Here's the drawing with two shaded views (mm, measured from the low corner). I have some questions. Give positions to 0.01 mm unless a question says otherwise; leave off trailing zeros. Loops run counter-clockwise (first coordinate to the right, second up) from the corner with the lowest first, then second, coordinate; pieces in that order, holes last. Notation, with made-up numbers: (-35, -34.5) - (6, -34.5) arc R20 cw to (6, -28.5) - close; hole circle Ø9 at (75, 30). An arc over 180 degrees is marked (long way). Use one line per item in the form item = value.
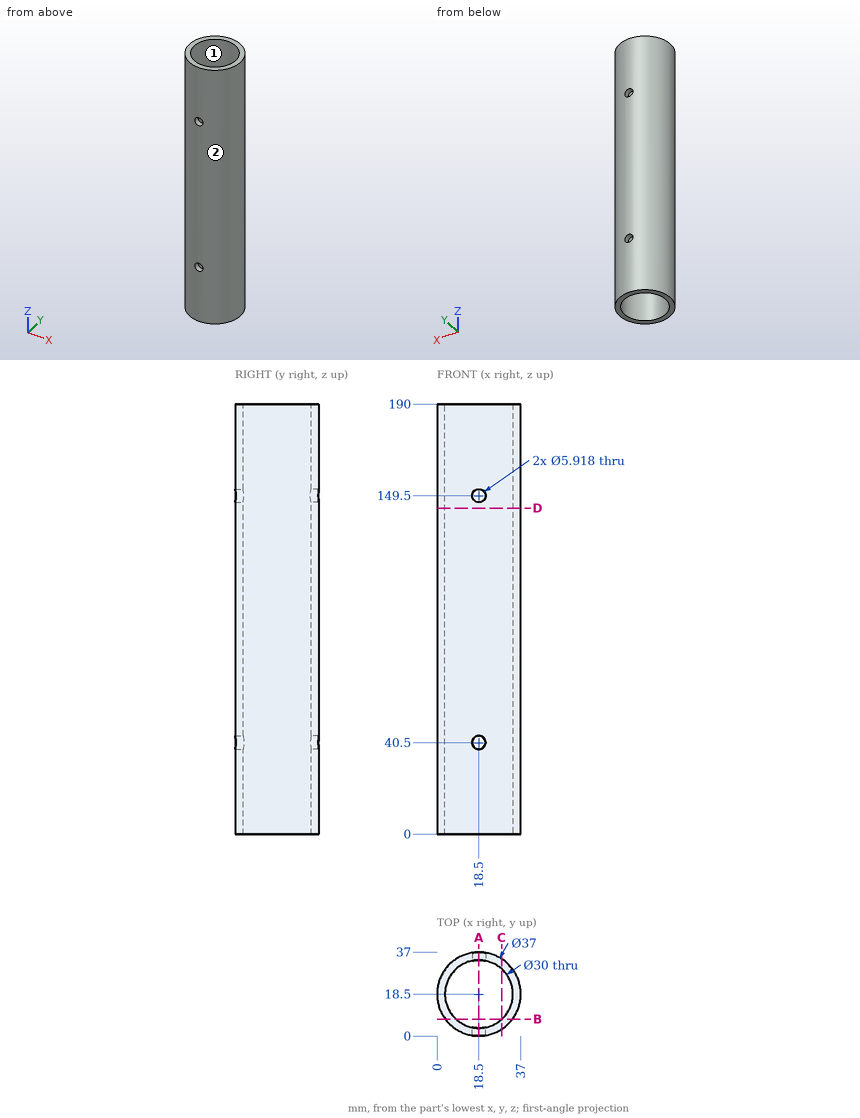
(1) Thinking about a two-plate mould opening in X: for the marked faces 1 and 2, which applies, pulls with the +X half, pulls with the -X half, needs draft (parallel to the pull), parting line crosses it, or undercut?
Geometry says:
face_1 = undercut
face_2 = parting line crosses it
(2) If I drill on probe 1 along Y at (x, z) = (30.5, 142.5); probe 2 along Y at (x, z) = (13, 171) (1 decimal); probe 3 along X at (y, z) = (8.5, 103.5) (1 decimal), over which ranges is the centre line in solid material (lowest first)?
Geometry says:
probe_1 = 4.42 to 9.5, 27.5 to 32.58
probe_2 = 0.8 to 4.5, 32.5 to 36.2
probe_3 = 2.9 to 7.3, 29.7 to 34.1
(3) If we section it at C-C (x = 28.5): List the corners of the cut face in (y, z) for me (1 decimal), plus the area to 3 significant figures.
Geometry says:
outline = (2.9, 0) - (7.3, 0) - (7.3, 190) - (2.9, 190) - close; (29.7, 0) - (34.1, 0) - (34.1, 190) - (29.7, 190) - close
area = 1,670 mm²
(4) If we section it at B-B (y = 7.5): List the corners of the cut face in (x, z) for me (1 decimal), plus the area to 3 significant figures.
Geometry says:
outline = (3.6, 0) - (8.3, 0) - (8.3, 190) - (3.6, 190) - close; (28.7, 0) - (33.4, 0) - (33.4, 190) - (28.7, 190) - close
area = 1,780 mm²
(5) For P1, Ø1.5, axis at y = 4, z = 138, coming from the -X side (1 decimal); P2, Ø8, axis at x = 31, z = 140, coming from the +Y side; P3, Ø6, axis at x = 14, z = 94, coming from the -Y side, each with a flat end and sliding along its axis, tell me the tip position at first contact or that it passes through.
Geometry says:
P1 = 6.1
P2 = 34.93
P3 = 0.06
(6) If we section it at A-A (x = 18.5): List the corners of the cut face in (y, z) for me.
Geometry says:
outline = (0, 0) - (3.5, 0) - (3.5, 37.54) - (0, 37.54) - close; (0, 43.46) - (3.5, 43.46) - (3.5, 146.54) - (0, 146.54) - close; (0, 152.46) - (3.5, 152.46) - (3.5, 190) - (0, 190) - close; (33.5, 0) - (37, 0) - (37, 37.54) - (33.5, 37.54) - close; (33.5, 43.46) - (37, 43.46) - (37, 146.54) - (33.5, 146.54) - close; (33.5, 152.46) - (37, 152.46) - (37, 190) - (33.5, 190) - close
(7) If we section it at D-D (z = 144): List the corners of the cut face in (x, y) for me.
Geometry says:
outline = circle Ø37 at (18.5, 18.5); hole circle Ø30 at (18.5, 18.5)
